Part model, mm, in its own coordinate system. A direction names the side the tool comes from. Give positions to 0.01 mm unless a question says otherwise; leave off trailing zeros. Write each loop counter-clockwise with the first axis right and the second up, starting at its lowest first coordinate (ties: lowest second). Pieces come first, ordered by that corner, then holes. Notation, with made-up numbers: M 14,34.5 L 22,34.5 A22 ccw 22,49.5 Z; hole C -18,43.25 d5. An arc over 180 degrees is marked long. Use CSV: the item, a comma, the result in double quotes. Start each with the question number.
1. Band-saw the part on B-B, the plane y = 58.35. Count the separate pieces of the cut face and the enclosed holes in it, then the cut area to 3 significant figures.
2. 3-axis set-ups, long thin cutter, end or side, ignore diameter. For faces 1 (the face through (16.8, 10.1, 4.6)), 2 (the face through (23, 7, 9)), 3 (the face through (36, 60, 3.2)): which of +Z, -Z, +X, -X, +Y, -Y reach the whole face in a straight line?
3. Band-saw the part on A-A, the plane x = 50. List the corners of the cut face in (y, z), then the cut area to 3 significant figures.
4. Drill centre lines: line 1 along X through (y, z) = (58.35, 1.25); line 2 along Y through (x, z) = (35.5, 8.25); line 3 along Y through (x, z) = (19, 6). Where is each one in solid material? Low to high. Write a range as from..to.
5. Mould opens along Y. For faces 4 (the face through (31.961, 60.297, 1.78)), 5 (the face through (0.801, 0.775, 14.886)), 6 (the face through (0.775, 63.199, 0.114)) say: pulls with the +Y half, pulls with the -Y half, needs draft (parallel to the pull), parting line crosses it, or undercut.
6. Drop flat-ended pins along their axis: pin 1 Ø10 at (x, y) = (40, 10) entering from +Z; pin 2 Ø7 at (x, y) = (60, 10) entering from -Z. Give the stop position or say it passes through.
from build123d import *

# Parameters (mm, degrees)
SKETCH_W        = 100
SKETCH_H        = 64
SKETCH_R        = 10.1
SKETCH_R_2      = 1.8
SKETCH_R_3      = 3.2
SKETCH_R_4      = 4
PAD_DEPTH       = 15
SKETCH001_R     = 11.2
SKETCH001_R_2   = 6
POCKET_DEPTH    = 6
SKETCH002_R     = 3.2
POCKET001_DEPTH = 3.2
SKETCH003_R     = 6
POCKET002_DEPTH = 6
SKETCH004_R     = 3.2
POCKET003_DEPTH = 15
FILLET_R        = 2
CHAMFER_SIZE    = 0.4
CHAMFER001_SIZE = 0.4


with BuildPart() as part:
    # Sketch → Pad (new body)
    with BuildSketch(Plane.XY):
        with Locations((50, 32)):
            Rectangle(SKETCH_W, SKETCH_H)
        with Locations((50, 42.85)):
            Circle(SKETCH_R, mode=Mode.SUBTRACT)
        with Locations((65.5, 58.35)):
            Circle(SKETCH_R_2, mode=Mode.SUBTRACT)
        with Locations((65.5, 27.35)):
            Circle(SKETCH_R_2, mode=Mode.SUBTRACT)
        with Locations((34.5, 27.35)):
            Circle(SKETCH_R_2, mode=Mode.SUBTRACT)
        with Locations((34.5, 58.35)):
            Circle(SKETCH_R_2, mode=Mode.SUBTRACT)
        with Locations((20, 10)):
            Circle(SKETCH_R_3, mode=Mode.SUBTRACT)
        with Locations((80, 10)):
            Circle(SKETCH_R_3, mode=Mode.SUBTRACT)
        with Locations((82, 42.85)):
            Circle(SKETCH_R_4, mode=Mode.SUBTRACT)
        with Locations((18, 42.85)):
            Circle(SKETCH_R_4, mode=Mode.SUBTRACT)
    extrude(amount=PAD_DEPTH)

    # Sketch001 (on Face15 of Pad) → Pocket (cut)
    with BuildSketch(Plane.XY.offset(15)):
        with Locations((50, 42.85)):
            Circle(SKETCH001_R)
        with Locations((20, 10)):
            Circle(SKETCH001_R_2)
        with Locations((80, 10)):
            Circle(SKETCH001_R_2)
    extrude(amount=-POCKET_DEPTH, mode=Mode.SUBTRACT)

    # Sketch002 (on Face4 of Pocket) → Pocket001 (cut)
    with BuildSketch(Plane(origin=(0, 0, 0), x_dir=(1, 0, 0), z_dir=(0, 0, -1))):
        with Locations((34.5, -27.35)):
            Circle(SKETCH002_R)
        with Locations((65.5, -27.35)):
            Circle(SKETCH002_R)
        with Locations((34.5, -58.35)):
            Circle(SKETCH002_R)
        with Locations((65.5, -58.35)):
            Circle(SKETCH002_R)
    extrude(amount=-POCKET001_DEPTH, mode=Mode.SUBTRACT)

    # Sketch003 (on Face5 of Pocket001) → Pocket002 (cut)
    with BuildSketch(Plane.XY.offset(15)):
        with Locations((40, 10)):
            Circle(SKETCH003_R)
        with Locations((60, 10)):
            Circle(SKETCH003_R)
    extrude(amount=-POCKET002_DEPTH, mode=Mode.SUBTRACT)

    # Sketch004 (on Face4 of Pocket002) → Pocket003 (cut)
    with BuildSketch(Plane(origin=(0, 0, 0), x_dir=(1, 0, 0), z_dir=(0, 0, -1))):
        with Locations((40, -10)):
            Circle(SKETCH004_R)
        with Locations((60, -10)):
            Circle(SKETCH004_R)
    extrude(amount=-POCKET003_DEPTH, mode=Mode.SUBTRACT)

    # Fillet
    fillet_edges = [part.edges().sort_by_distance(p)[0] for p in [
        (0, 64, 7.5),
        (100, 64, 7.5),
        (100, 0, 7.5),
        (0, 0, 7.5),
    ]]
    fillet(fillet_edges, radius=FILLET_R)

    # Chamfer
    chamfer_edges = [part.edges().sort_by_distance(p)[0] for p in [
        (50, 64, 15),
        (0.585786, 63.414214, 15),
        (99.414214, 63.414214, 15),
        (0, 32, 15),
        (100, 32, 15),
        (0.585786, 0.585786, 15),
        (99.414214, 0.585786, 15),
        (50, 0, 15),
        (74, 10, 15),
        (54, 10, 15),
        (63.7, 27.35, 15),
        (34, 10, 15),
        (14, 10, 15),
        (32.7, 27.35, 15),
        (78, 42.85, 15),
        (63.7, 58.35, 15),
        (38.8, 42.85, 15),
        (14, 42.85, 15),
        (32.7, 58.35, 15),
    ]]
    chamfer(chamfer_edges, length=CHAMFER_SIZE)

    # Chamfer001
    chamfer001_edges = [part.edges().sort_by_distance(p)[0] for p in [
        (50, 64, 0),
        (0.585786, 63.414214, 0),
        (99.414214, 63.414214, 0),
        (0, 32, 0),
        (100, 32, 0),
        (0.585786, 0.585786, 0),
        (99.414214, 0.585786, 0),
        (50, 0, 0),
        (76.8, 10, 0),
        (56.8, 10, 0),
        (62.3, 27.35, 0),
        (36.8, 10, 0),
        (16.8, 10, 0),
        (31.3, 27.35, 0),
        (78, 42.85, 0),
        (62.3, 58.35, 0),
        (39.9, 42.85, 0),
        (14, 42.85, 0),
        (31.3, 58.35, 0),
    ]]
    chamfer(chamfer001_edges, length=CHAMFER001_SIZE)


solid = part.part
Output:
1,separate pieces,"3"
1,enclosed holes,"0"
1,area,"1,370 mm²"
2,face 1,"+Z, -Z"
2,face 2,"+Z"
2,face 3,"-Z"
3,outline,"M 0,0.4 L 0.4,0 L 32.35,0 L 32.75,0.4 L 32.75,9 L 31.65,9 L 31.65,14.6 L 31.25,15 L 0.4,15 L 0,14.6 Z; M 52.95,0.4 L 53.35,0 L 63.6,0 L 64,0.4 L 64,14.6 L 63.6,15 L 54.45,15 L 54.05,14.6 L 54.05,9 L 52.95,9 Z"
3,area,"643 mm²"
4,line 1,"x = 0..31.3, 37.7..62.3, 68.7..100"
4,line 2,"y = 0..25.85, 28.85..56.85, 59.85..64"
4,line 3,"y = 0..6.96, 13.04..38.98, 46.72..64"
5,face 4,"undercut"
5,face 5,"pulls with the -Y half"
5,face 6,"pulls with the +Y half"
6,pin 1,"stops at z = 9"
6,pin 2,"stops at z = 0.1"
